from build123d import *

# Parameters (mm, degrees)
F1_DEPTH = 40
F2_T     = -4


with BuildPart() as f1:
    # F0 (on Front) → F1 (new body)
    with BuildSketch(Plane.XZ):
        with BuildLine():
            Line((44.70779, 0), (-45.29221, 0))
            ThreePointArc((-45.29221, 0), (-0.29221, -45), (44.70779, 0))
        make_face()
    extrude(amount=F1_DEPTH)

    # F2
    f2_openings = [f1.faces().sort_by_distance(p)[0] for p in [
        (-0.29221, -20, 0),
    ]]
    offset(amount=F2_T, openings=f2_openings)


solid = f1.part
The model under review builds one solid part; all positions refer to its coordinate system, in mm. A direction names the side the tool comes from. Coordinates: 2 decimals unless noted, no trailing zeros. Loops run counter-clockwise (first coordinate to the right, second up) from the corner with the lowest first, then second, coordinate; pieces in that order, holes last.
(1) Consider section A-A, the plane z = -21. Give the boundary of the cut face in (x, y).
Determined:
outline: (-40.09, -40) - (39.51, -40) - (39.51, 0) - (-40.09, 0) - close; hole (-35.51, -36) - (34.92, -36) - (34.92, -4) - (-35.51, -4) - close
(2) Consider section C-C, the plane y = -28.5. Give the boundary of the cut face in (x, z).
Determined:
outline: (-45.29, 0) arc R45 ccw to (44.71, 0) - (40.71, 0) arc R41 cw to (-41.29, 0) - close
(3) Consider section B-B, the plane x = 18. Give the boundary of the cut face in (y, z).
Determined:
outline: (-40, -41.11) - (0, -41.11) - (0, 0) - (-4, 0) - (-4, -36.69) - (-36, -36.69) - (-36, 0) - (-40, 0) - close
(4) Tool access review of faces 1 (the flat face through (-1, -36, -16)), 2 (the flat face through (-1, -40, -17)): name each direction out of +Z, -Z, +X, -X, +Y, -Y from which nothing blocks a thin tool from reaching the whole face with its end or side.
Determined:
face 1: +Z
face 2: +Z, -Z, +X, -X, -Y
(5) Insertion check: P1, Ø12, axis at y = -8.5, z = -39, coming from the -X side; P2, Ø5, axis at y = -11, z = -19.5, coming from the -X side; P3, Ø5, axis at x = -2, y = -4.5, coming from the -Z side. Each pin has a flat end and moves straight along its axis. Give the tip position at first contact, or say it passes through.
Determined:
P1: stops at x = -30.89
P2: stops at x = -41.96
P3: stops at z = -45
(6) Consider section D-D, the plane z = -40. Give the boundary of the cut face in (x, y).
Determined:
outline: (-20.91, -40) - (20.32, -40) - (20.32, 0) - (-20.91, 0) - close; hole (-9.29, -36) - (8.71, -36) - (8.71, -4) - (-9.29, -4) - close
(7) Draft analysis for pull direction X (two halves, no side actions). For faces 3 (the cylindrical face through (-1.19, -19.78, -40.99)), 4 (the cylindrical face through (-1.28, -19.72, -44.99)), 5 (the flat face through (-1, 0, -17)), state which applies: +X half, -X half, draft (parallel to the pull), parting line (faces both ways), or undercut.
Determined:
face 3: undercut
face 4: parting line
face 5: draft
(8) Wall thickness on L1, parallel to Y at x = 24.5, z = -23; L2, parallel to X at y = -7, z = -17.5; L3, parallel to X at y = -12, z = -1.5: over which ranges is each line inside the solid? List them lowest first.
Determined:
L1: y = -40 to -36, -4 to 0
L2: x = -41.75 to -37.37, 36.79 to 41.17
L3: x = -45.27 to -41.26, 40.68 to 44.68
